from build123d import *

# Parameters (mm, degrees)
F1_DEPTH  = 6.35
F2_W      = 5.715
F2_H      = 16.8021
F3_DEPTH  = 33.011516
F4_W      = 3.99288
F4_H      = 5.715
F5_DEPTH  = 68.7705
F6_W      = 0.3175
F6_H      = 138.176
F7_DEPTH  = 63.5
F9_DEPTH  = 25.4
F10_W     = 6.0325
F10_H     = 18.3896
F11_DEPTH = 67.49388
F13_DEPTH = 0.3175
F14_W     = 0.3175
F14_H     = 17.1196
F15_DEPTH = 6.0325


with BuildPart() as f1:
    # F0 (on Front) → F1 (new body)
    with BuildSketch(Plane.XZ):
        Polygon((-33.528, 69.088), (-33.528, -69.088), (33.130033, -69.088), (33.130033, -51.9684), (-29.21762, -51.9684), (-29.21762, 60.152978), (-29.21762, 69.088), align=None)
    extrude(amount=F1_DEPTH)

    # F2 (on Right) → F3 (cut, symmetric)
    with BuildSketch(Plane.YZ):
        with Locations((-3.175, 60.36945)):
            Rectangle(F2_W, F2_H)
        with Locations((-3.175, -60.36945)):
            Rectangle(F2_W, F2_H)
    extrude(amount=F3_DEPTH, both=True, mode=Mode.SUBTRACT)

    # F4 (on Top) → F5 (cut, symmetric)
    with BuildSketch(Plane.XY):
        with Locations((-31.21406, -3.175)):
            Rectangle(F4_W, F4_H)
    extrude(amount=F5_DEPTH, both=True, mode=Mode.SUBTRACT)

    # F6 (on face) → F7 (join)
    with BuildSketch(Plane.YZ.offset(-29.21762)):
        with Locations((-0.15875, 0)):
            Rectangle(F6_W, F6_H)
    extrude(amount=F7_DEPTH)

    # F8 (on face) → F9 (cut)
    with BuildSketch(Plane.YZ.offset(33.130033)):
        Polygon((-6.0325, -51.9684), (-6.0325, -68.7705), (-0.3175, -68.7705), (-0.3175, -52.373883), (-0.3175, -51.9684), align=None)
    extrude(amount=-F9_DEPTH, mode=Mode.SUBTRACT)

    # F10 (on face) → F11 (cut, through all)
    with BuildSketch(Plane.YZ.offset(-33.2105)):
        with Locations((-3.33375, 61.1632)):
            Rectangle(F10_W, F10_H)
    extrude(amount=F11_DEPTH, mode=Mode.SUBTRACT)

    # F12 (on face) → F13 (cut)
    with BuildSketch(Plane(origin=(0, 0, 0), x_dir=(-1, 0, 0), z_dir=(0, 1, 0))):
        Polygon((33.528, 69.088), (-34.28238, 69.088), (-34.28238, -69.088), (-33.130033, -69.088), align=None)
    extrude(amount=-F13_DEPTH, mode=Mode.SUBTRACT)

    # F14 (on face) → F15 (cut, through all)
    with BuildSketch(Plane.XZ.offset(6.35)):
        with Locations((32.971283, -60.5282)):
            Rectangle(F14_W, F14_H)
    extrude(amount=-F15_DEPTH, mode=Mode.SUBTRACT)


solid = f1.part
Build history of the part. All positions in model axes, mm. A direction names the side the tool comes from. Coordinates: 2 decimals unless noted, no trailing zeros. Write each loop counter-clockwise with the first axis right and the second up, starting at its lowest first coordinate (ties: lowest second). Pieces come first, ordered by that corner, then holes.
(1) Cut at B-B on z = 8. List the corners of the cut face in (x, y).
(2) Drill centre lines: line 1 (X direction, y = -6, z = 60); line 2 (Z direction, x = -20.5, y = -2.75); line 3 (Y direction, x = -8, z = -41). Where is each one in solid material? Low to high.
(3) Pin check, flat tips, straight feed: pin 1 Ø20 at (x, z) = (4, -29.5) entering from -Y; pin 2 Ø1 at (x, y) = (22, -2) entering from +Z; pin 3 Ø1 at (y, z) = (-3.5, -8.5) entering from +X. Stop position of each tip, or through.
(4) Cut at C-C on x = 14.5. List the corners of the cut face in (y, z), and give its area (3 significant figures).
(5) Cut at A-A on y = -4.75. List the corners of the cut face in (x, z).
(6) 3-axis set-ups, long thin cutter, end or side, ignore diameter. For faces 5 (the flat face through (0, -3, -68.77)), 6 (the flat face through (-1, -3, -69.088)): which of +Z, -Z, +X, -X, +Y, -Y reach the whole face in a straight line?
(7) Mould opens along Y. For faces 1 (the flat face through (-33.21, -3, 1)), 2 (the flat face through (-10, -6.35, -56)), 3 (the flat face through (-15, 0, -30)), 4 (the flat face through (-15, -0.317, -30)) say: pulls with the +Y half, pulls with the -Y half, needs draft (parallel to the pull), parting line crosses it, or undercut.
Working result:
1. outline: (-33.53, -6.35) - (-29.22, -6.35) - (-29.22, -6.03) - (-33.21, -6.03) - (-33.21, -0.32) - (-4.06, -0.32) - (-4.06, 0) - (-33.53, 0) - close
2. line 1: x = -33.53 to -33.21
2. line 2: z = -69.09 to -68.77
2. line 3: y = -0.32 to 0
3. pin 1: stops at y = -0.32
3. pin 2: stops at z = -68.77
3. pin 3: stops at x = -33.21
4. outline: (-6.35, -69.09) - (0, -69.09) - (0, -30.47) - (-0.32, -30.47) - (-0.32, -68.77) - (-6.03, -68.77) - (-6.03, -51.97) - (-6.35, -51.97) - close
4. area: 19.5 mm2
5. outline: (-33.53, -69.09) - (32.81, -69.09) - (32.81, -68.77) - (-33.21, -68.77) - (-33.21, 69.09) - (-33.53, 69.09) - close
6. face 5: +Z, +X
6. face 6: -Z, +X, -X, +Y, -Y
7. face 1: undercut
7. face 2: pulls with the -Y half
7. face 3: pulls with the +Y half
7. face 4: undercut
